Here's how the part is built. I have some questions about the finished solid (model axes, mm). Give positions to 0.01 mm unless a question says otherwise; leave off trailing zeros. Loops run counter-clockwise (first coordinate to the right, second up) from the corner with the lowest first, then second, coordinate; pieces in that order, holes last.
Q1. If we section it at A-A (x = -144): Please give me the cut outline in (y, z), plus the area to 3 significant figures.
Q2. I need wall thicknesses on line 1 (Y direction, x = -104.5, z = 2.25); line 2 (Y direction, x = -104, z = 1); line 3 (Y direction, x = -78, z = 3). Which ranges of each line are inside material? Lowest first, please.
Q3. Will these pins go through, and if not, where does the flat tip stop? P1, Ø3, axis at x = -103.91, y = 36.11, coming from the +Z side; P2, Ø5, axis at x = -109.98, y = 2.23, coming from the -Z side; P3, Ø5, axis at x = -142, z = 7, coming from the -Y side; P4, Ø3, axis at y = 67, z = 2, coming from the +X side.
Q4. If we section it at C-C (y = -36.5): Please give me the cut outline in (x, z).
Q5. If we section it at D-D (x = -119): Please give me the cut outline in (y, z).
Q6. If we section it at B-B (z = 4): Give the number of separate pieces and of enclosed holes in the cut face, plus the area to 3 significant figures.
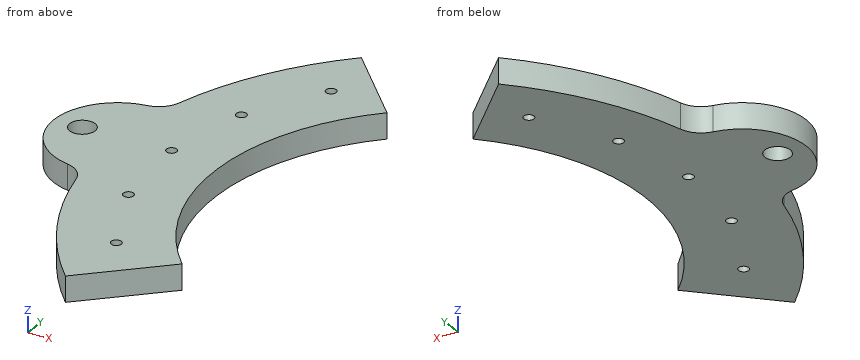
from build123d import *

# Parameters (mm, degrees)
SKETCH2_R           = 5
BOSS_EXTRUDE1_DEPTH = 10
FILLET1_R           = 10
SKETCH3_R           = 2
CUT_EXTRUDE1_DEPTH  = 181.48545662


with BuildPart() as part:
    # Sketch2 → Boss-Extrude1 (new body)
    with BuildSketch(Plane.XY):
        with BuildLine():
            Line((-63.639610307, 63.639610307), (-91.923881554, 91.923881554))
            ThreePointArc((-91.923881554, 91.923881554), (-114.764290969, 61.066828299), (-127.596153846, 24.884162105))
            ThreePointArc((-127.596153846, 24.884162105), (-155, 0), (-127.596153846, -24.884162105))
            ThreePointArc((-127.596153846, -24.884162105), (-114.764290969, -61.066828299), (-91.923881554, -91.923881554))
            Line((-91.923881554, -91.923881554), (-63.639610307, -63.639610307))
            ThreePointArc((-63.639610307, -63.639610307), (-90, 0), (-63.639610307, 63.639610307))
        make_face()
        with Locations((-144, 0)):
            Circle(SKETCH2_R, mode=Mode.SUBTRACT)
    extrude(amount=BOSS_EXTRUDE1_DEPTH)

    # Fillet1
    fillet1_edges = [part.edges().sort_by_distance(p)[0] for p in [
        (-127.596153846, -24.884162105, 5),
        (-127.596153846, 24.884162105, 5),
    ]]
    fillet(fillet1_edges, radius=FILLET1_R)

    # Sketch3 → Cut-Extrude1 (cut, through all)
    with BuildSketch(Plane.XY.offset(10)):
        with Locations((-87.661776755, 66.448573319)):
            Circle(SKETCH3_R)
        with Locations((-103.90504242, 36.107369879)):
            Circle(SKETCH3_R)
        with Locations((-109.977358585, 2.231725501)):
            Circle(SKETCH3_R)
        with Locations((-105.284324634, -31.862375719)):
            Circle(SKETCH3_R)
        with Locations((-90.285327428, -62.837565605)):
            Circle(SKETCH3_R)
    extrude(amount=-CUT_EXTRUDE1_DEPTH, mode=Mode.SUBTRACT)


solid = part.part
Check sheet entries:
1. outline: (-20.71, 0) - (-5, 0) - (-5, 10) - (-20.71, 10) - close; (5, 0) - (20.71, 0) - (20.71, 10) - (5, 10) - close
1. area: 314 mm2
2. line 1: y = -77.33 to -33.7, -30.02 to 34.2, 38.02 to 77.33
2. line 2: y = -78 to -33.4, -30.33 to 34.11, 38.11 to 78
2. line 3: y = -78 to -44.9, 44.9 to 78
3. P1: passes through
3. P2: stops at z = 0
3. P3: stops at y = -23.12
3. P4: stops at x = -65.5
4. outline: (-124.77, 0) - (-82.27, 0) - (-82.27, 10) - (-124.77, 10) - close
5. outline: (-52.34, 0) - (52.34, 0) - (52.34, 10) - (-52.34, 10) - close
6. separate pieces: 1
6. enclosed holes: 6
6. area: 7,810 mm2
